```python
from build123d import *

# Parameters (mm, degrees)
BOSS_EXTRUDE1_DEPTH = 29.5
SKETCH4_W           = 50
SKETCH4_H           = 35
CUT_EXTRUDE1_DEPTH  = 68
SKETCH5_W           = 15.381078853
SKETCH5_H           = 2.6
CUT_EXTRUDE2_DEPTH  = 2


with BuildPart() as part:
    # Sketch1 → Boss-Extrude1 (new body)
    with BuildSketch(Plane.XY):
        Polygon((-22.49, 37.442535728), (-20.79, 38.235869061), (-19.35, 37.563869061), (-19.35, 26.640292624), (-20.79, 25.968292624), (-22.49, 26.761625958), align=None)
    extrude(amount=-BOSS_EXTRUDE1_DEPTH)

    # Sketch3 → Revolve1 (revolve)
    with BuildSketch(Plane(origin=(0, 32.102080843, 0), x_dir=(-1, 0, 0), z_dir=(0, -1, 0)), mode=Mode.PRIVATE) as revolve1_sk:
        with BuildLine():
            Line((22.49, 29.5), (40.49, 29.5))
            ThreePointArc((40.49, 29.5), (37.113405562, 13.37358399), (27.49, 0))
            Line((27.49, 0), (22.49, 0))
            Line((22.49, 0), (22.49, 29.5))
        make_face()
        with BuildLine():
            Line((23.79, 28.2), (39.171078853, 28.2))
            ThreePointArc((39.171078853, 28.2), (35.761046656, 13.533638438), (26.982175907, 1.3))
            Line((26.982175907, 1.3), (23.79, 1.3))
            Line((23.79, 1.3), (23.79, 28.2))
        make_face(mode=Mode.SUBTRACT)
    revolve(revolve1_sk.sketch.rotate(Axis((-22.49, 32.102080843, -29.5), (-1, 0, 0)), 90), axis=Axis((-22.49, 32.102080843, -29.5), (-1, 0, 0)))

    # Sketch4 → Cut-Extrude1 (cut)
    with BuildSketch(Plane(origin=(0, 0, 0), x_dir=(1, 0, 0), z_dir=(0, 1, 0))):
        with Locations((-35.281230145, 47)):
            Rectangle(SKETCH4_W, SKETCH4_H)
    extrude(amount=CUT_EXTRUDE1_DEPTH, mode=Mode.SUBTRACT)

    # Sketch5 → Cut-Extrude2 (cut)
    with BuildSketch(Plane(origin=(0, 0, -29.5), x_dir=(-1, 0, 0), z_dir=(0, 0, -1))):
        with Locations((31.480539427, 32.102080843)):
            Rectangle(SKETCH5_W, SKETCH5_H)
    extrude(amount=-CUT_EXTRUDE2_DEPTH, mode=Mode.SUBTRACT)


solid = part.part
```
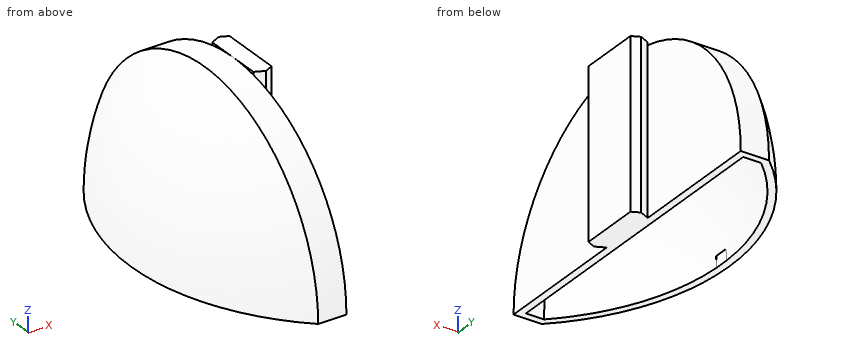
Check sheet for the modelled part. Datum: model origin and axes. Units: mm. Round coordinates to 2 decimals unless told otherwise and drop trailing zeros. Order: outer loops, then holes, each group sorted by start corner. A loop starts at its lowest first (then second) coordinate and runs counter-clockwise, first axis right, second up. Notation, with made-up numbers: (-35.75, 68) - (-11.75, 68) arc R23 ccw to (-11.75, 102) - close; hole circle Ø11 at (57.5, -32.75). An arc over 180 degrees is marked (long way). Answer as CSV lines item,"result". Start each with the question number.
1) Section check A-A (x = -26.25). Record the cut outline in (y, z).
2) Scan lines: probe 1 along X at (y, z) = (53, -19.75); probe 2 along X at (y, z) = (53, -25.5); probe 3 along Y at (x, z) = (-33, -18.75). Record each from-to range of solid material in increasing order.
3) Depth check by flat-ended pin: pin 1 (10 mm diameter, centred on y = 18.5, z = -11, fed in from -X); pin 2 (7 mm diameter, centred on y = 11, z = -8.5, fed in from +X); pin 3 (8.5 mm diameter, centred on y = 33.5, z = -19, fed in from -X); pin 4 (1 mm diameter, centred on x = -24, y = 9.5, fed in from -Z). Enter the tip coordinate at first touch or a pass-through.
Determined:
1,outline,"(2.6, -29.5) - (3.9, -29.5) arc R28.2 cw to (60.3, -29.5) - (61.6, -29.5) arc R29.5 ccw to start"
2,probe 1,"-33.19 to -31.58, -23.79 to -22.49"
2,probe 2,"-34.38 to -32.83, -23.79 to -22.49"
2,probe 3,"11.41 to 14.04, 50.16 to 52.8"
3,pin 1,"x = -36.25"
3,pin 2,"x = -22.49"
3,pin 3,"x = -40"
3,pin 4,"z = -29.5"
